```python
from build123d import *

# Parameters (mm, degrees)
FILLET1_R = 0.254


with BuildPart() as part:
    # Sketch2 → Revolve1 (revolve)
    with BuildSketch(Plane.XY):
        with BuildLine():
            Line((-12.7, 0), (-12.7, 10.795))
            ThreePointArc((-12.7, 10.795), (-12.142038418, 12.142038418), (-10.795, 12.7))
            Line((-10.795, 12.7), (-6.35, 12.7))
            Line((-6.35, 12.7), (-6.35, 6.35))
            Line((-6.35, 6.35), (-2.778125, 6.35))
            Line((-2.778125, 6.35), (-2.778125, 0))
            Line((-2.778125, 0), (-12.7, 0))
        make_face()
    revolve(axis=Axis((0, 0, 0), (0, 1, 0)))

    # Fillet1
    fillet1_edges = [part.edges().sort_by_distance(p)[0] for p in [
        (6.35, 12.7, 0),
    ]]
    fillet(fillet1_edges, radius=FILLET1_R)


solid = part.part
```
Part model, mm, in its own coordinate system. A direction names the side the tool comes from. Round coordinates to 2 decimals unless told otherwise and drop trailing zeros. Write each loop counter-clockwise with the first axis right and the second up, starting at its lowest first coordinate (ties: lowest second). Pieces come first, ordered by that corner, then holes. Notation, with made-up numbers: (-36.75, 61) -> (-8.75, 61) arc R13 cw to (-8.75, 67) -> close; hole circle Ø5 at (-29, 81.25). An arc over 180 degrees is marked (long way). Return JSON: item names as keys, results as strings. Group by question number.
Q1. Saw through at D-D on y = 8. Write the cut outline in (x, z).
Q2. Saw through at B-B on x = 0. Write the cut outline in (y, z) (3 decimals).
Q3. Which spindle directions (+Z, -Z, +X, -X, +Y, -Y) get a long thin tool onto all of the face, cutting with end or side? Do faces 4 (the cylindrical face through (1.38, 9.36, -6.2)), 5 (the flat face through (-5, 12.7, 5)). Say none if no direction does.
Q4. Saw through at A-A on z = 0. Write the cut outline in (x, y) (3 decimals).
Q5. Mould opens along Z. For faces 1 (the cylindrical face through (2.75, 5.47, -12.4)), 2 (the cylindrical face through (-2.65, 3.13, 0.83)), 3 (the flat face through (0, 0, 3)) say: pulls with the +Z half, pulls with the -Z half, needs draft (parallel to the pull), parting line crosses it, or undercut.
Q6. Saw through at C-C on y = 5. Write the cut outline in (x, z), plus the area to 3 significant figures.
Q7. Probe L1, parallel to X at y = 7, z = 0.25; L2, parallel to Z at x = 0, y = 3.25. List the from-to ranges inside material, lowest first. Write a range as [from, to].
Q8. Pin check, flat tips, straight feed: pin 1 (3 mm diameter, centred on x = -8.5, y = 5.5, fed in from -Z); pin 2 (6 mm diameter, centred on y = 10.5, z = 5, fed in from -X); pin 3 (4 mm diameter, centred on x = -2, z = -0.5, fed in from +Y); pin 4 (4.5 mm diameter, centred on x = 0, z = 0, fed in from +Y). Stop position of each tip, or through.
Answer:
{
 "1": {"outline": "circle Ø25.4 at (0, 0); hole circle Ø12.7 at (0, 0)"},
 "2": {"outline": "(0, -12.7) -> (10.795, -12.7) arc R1.905 ccw to (12.7, -10.795) -> (12.7, -6.604) arc R0.254 ccw to (12.446, -6.35) -> (6.35, -6.35) -> (6.35, -2.778) -> (0, -2.778) -> close; (0, 2.778) -> (6.35, 2.778) -> (6.35, 6.35) -> (12.446, 6.35) arc R0.254 ccw to (12.7, 6.604) -> (12.7, 10.795) arc R1.905 ccw to (10.795, 12.7) -> (0, 12.7) -> close"},
 "3": {"face 4": "+Y", "face 5": "+Z, -Z, +X, -X, +Y"},
 "4": {"outline": "(-12.7, 0) -> (-2.778, 0) -> (-2.778, 6.35) -> (-6.35, 6.35) -> (-6.35, 12.446) arc R0.254 ccw to (-6.604, 12.7) -> (-10.795, 12.7) arc R1.905 ccw to (-12.7, 10.795) -> close; (2.778, 0) -> (12.7, 0) -> (12.7, 10.795) arc R1.905 ccw to (10.795, 12.7) -> (6.604, 12.7) arc R0.254 ccw to (6.35, 12.446) -> (6.35, 6.35) -> (2.778, 6.35) -> close"},
 "5": {"face 1": "parting line crosses it", "face 2": "undercut", "face 3": "needs draft"},
 "6": {"outline": "circle Ø25.4 at (0, 0); hole circle Ø5.56 at (0, 0)", "area": "482 mm2"},
 "7": {"L1": "[-12.7, -6.35], [6.35, 12.7]", "L2": "[-12.7, -2.78], [2.78, 12.7]"},
 "8": {"pin 1": "z = -10.6", "pin 2": "x = -12.54", "pin 3": "y = 6.35", "pin 4": "through"}
}
